Could you check a few things on this model? Use its own coordinates, in mm. Face numbers are marked on the shaded views. Give positions to 0.01 mm unless a question says otherwise; leave off trailing zeros. Loops run counter-clockwise (first coordinate to the right, second up) from the corner with the lowest first, then second, coordinate; pieces in that order, holes last. Notation, with made-up numbers: M 24,31.5 L 49,31.5 A27 cw 49,63.5 Z; hole C 38,-33.5 d10. An arc over 180 degrees is marked long. Use CSV: the item, a comma, the result in double quotes.
```python
from build123d import *

# Parameters (mm, degrees)
BOSS_EXTRU_1_DEPTH = 30
D_GAGEMENT_M31_D   = 3.4
D_GAGEMENT_M32_D   = 3.4


with BuildPart() as part:
    # Esquisse1 → Boss.-Extru.1 (new body)
    with BuildSketch(Plane.XY):
        with BuildLine():
            Line((22.5, 63), (-22.5, 63))
            Line((-22.5, 63), (-39.909502262, 48.746606335))
            ThreePointArc((-39.909502262, 48.746606335), (-56.050152659, 28.764220604), (-62.872887638, 4))
            Line((-62.872887638, 4), (-71, 4))
            Line((-71, 4), (-71, 0))
            Line((-71, 0), (-59, 0))
            ThreePointArc((-59, 0), (0, 59), (59, 0))
            Line((59, 0), (71, 0))
            Line((71, 0), (71, 4))
            Line((71, 4), (62.872887638, 4))
            ThreePointArc((62.872887638, 4), (56.050152659, 28.764220604), (39.909502262, 48.746606335))
            Line((39.909502262, 48.746606335), (22.5, 63))
        make_face()
    extrude(amount=BOSS_EXTRU_1_DEPTH)

    # Dégagement M31 (through all)
    with Locations(Plane(origin=(0, 4, 0), x_dir=(1, 0, 0), z_dir=(0, 1, 0))):
        with Locations((-67, -25), (-67, -5), (67, -25), (67, -5)):
            Hole(D_GAGEMENT_M31_D / 2)

    # Dégagement M32 (through all)
    with Locations(Plane(origin=(0, 63, 0), x_dir=(1, 0, 0), z_dir=(0, 1, 0))):
        with Locations((20, -5), (-20, -5), (-20, -25), (20, -25)):
            Hole(D_GAGEMENT_M32_D / 2)


solid = part.part
```
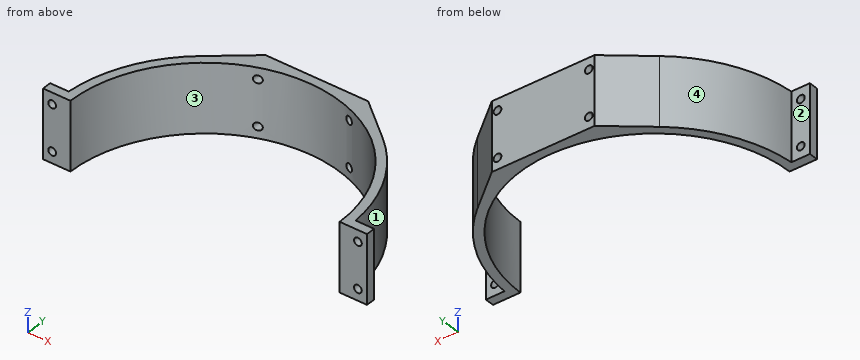
1. If we mould it in two halves opening along X, with no side actions, what happens to the marked faces 1, 2, 3 and 4? For each: +X half, -X half, draft (parallel to the pull), parting line (faces both ways), or undercut.
Outcome:
face 1,"+X half"
face 2,"draft"
face 3,"undercut"
face 4,"-X half"
2. Please list where these lines run through material, in increasing order: line 1 (Z direction, x = 67, y = 1.3); line 2 (X direction, y = 1, z = 5); line 3 (X direction, y = 59.75, z = 25).
Outcome:
line 1,"0 to 3.3, 6.7 to 23.3, 26.7 to 30"
line 2,"-71 to -68.7, -65.3 to -58.99, 58.99 to 65.3, 68.7 to 71"
line 3,"-26.47 to -21.7, -18.3 to 18.3, 21.7 to 26.47"
3. I want a section at B-B, the plane y = 57.5. List the corners of the cut face in (x, z) for me.
Outcome:
outline,"M -29.22,0 L -13.22,0 L -13.22,30 L -29.22,30 Z; M 13.22,0 L 29.22,0 L 29.22,30 L 13.22,30 Z; hole C -20,5 d3.4; hole C -20,25 d3.4; hole C 20,5 d3.4; hole C 20,25 d3.4"
4. I'm going to push flat-ended pins straight in: pin 1 Ø12 at (x, z) = (38.5, 8) entering from +Y; pin 2 Ø5.5 at (x, z) = (20, 25) entering from -Y; pin 3 Ø12 at (x, z) = (0.5, 7.5) entering from -Y; pin 4 Ø3 at (x, z) = (-20, 25) entering from +Y. Where does each tip first touch, or does it pass through?
Outcome:
pin 1,"y = 54.81"
pin 2,"y = 54.44"
pin 3,"y = 58.64"
pin 4,"through"
5. I want a section at A-A, the plane x = -67. List the corners of the cut face in (y, z) for me, then the cut area to 3 significant figures.
Outcome:
outline,"M 0,0 L 4,0 L 4,3.3 L 0,3.3 Z; M 0,6.7 L 4,6.7 L 4,23.3 L 0,23.3 Z; M 0,26.7 L 4,26.7 L 4,30 L 0,30 Z"
area,"92.8 mm2"
6. I want a section at C-C, the plane z = 25. List the corners of the cut face in (x, y) for me.
Outcome:
outline,"M -71,0 L -68.7,0 L -68.7,4 L -71,4 Z; M -65.3,0 L -59,0 A59 cw -21.7,54.86 L -21.7,63 L -22.5,63 L -39.91,48.75 A63 ccw -62.87,4 L -65.3,4 Z; M -18.3,56.09 A59 cw 18.3,56.09 L 18.3,63 L -18.3,63 Z; M 21.7,54.86 A59 cw 59,0 L 65.3,0 L 65.3,4 L 62.87,4 A63 ccw 39.91,48.75 L 22.5,63 L 21.7,63 Z; M 68.7,0 L 71,0 L 71,4 L 68.7,4 Z"
7. I want a section at D-D, the plane y = 51. List the corners of the cut face in (x, z) for me, then the cut area to 3 significant figures.
Outcome:
outline,"M -37.16,0 L -29.66,0 L -29.66,30 L -37.16,30 Z; M 29.66,0 L 37.16,0 L 37.16,30 L 29.66,30 Z"
area,"450 mm2"
